from build123d import *

# Parameters (mm, degrees)
F0_R     = 16
F1_DEPTH = 16
F1_TAPER = 1
F2_R     = 16
F3_DEPTH = 16
F4_R     = 2.5
F5_DEPTH = 5
F7_R     = 4.75
F8_DEPTH = 1.5


with BuildPart() as f1:
    # F0 (on Top) → F1 (new body)
    with BuildSketch(Plane.XY):
        Circle(F0_R)
    extrude(amount=F1_DEPTH, taper=F1_TAPER)

    # F2 (on Front) → F3 (cut, symmetric)
    with BuildSketch(Plane.XZ):
        with Locations((0, 20)):
            Circle(F2_R)
    extrude(amount=F3_DEPTH, both=True, mode=Mode.SUBTRACT)

    # F4 (on face) → F5 (cut)
    with BuildSketch(Plane(origin=(0, 0, 0), x_dir=(1, 0, 0), z_dir=(0, 0, -1))):
        Circle(F4_R)
    extrude(amount=-F5_DEPTH, mode=Mode.SUBTRACT)

    # F7 (on offset) → F8 (cut)
    with BuildSketch(Plane.XY.offset(5)):
        Circle(F7_R)
    extrude(amount=-F8_DEPTH, mode=Mode.SUBTRACT)


solid = f1.part
Work out the finished part from the listing and answer in its coordinate system (mm). A direction names the side the tool comes from. Give positions to 0.01 mm unless a question says otherwise; leave off trailing zeros. Order: outer loops, then holes, each group sorted by start corner. A loop starts at its lowest first (then second) coordinate and runs counter-clockwise, first axis right, second up. Notation, with made-up numbers: (60.25, 29) -> (77.25, 29) arc R16 cw to (77.25, 48) -> close; hole circle Ø4 at (-16.75, -1). An arc over 180 degrees is marked (long way). One line per item, written item: value.
Item 1: Flat-ended cylindrical pins translate along their axes: P1, Ø8, axis at x = 11.5, z = 2.5, coming from the -Y side; P2, Ø12, axis at x = 4, y = -7.5, coming from the +Z side; P3, Ø6, axis at x = 8, y = -8, coming from the +Z side. Find the tip coordinate at first contact, or state that the pin passes through.
Answer sheet:
P1: y = -14.09
P2: z = 7.51
P3: z = 8.38
Item 2: A tool of negligible diameter and unlimited length cuts with its end or side. For faces 1 (the flat face through (2, -2, 3.5)), 2 (the cylindrical face through (-4.9, -0.22, 4.77)), from which of +Z, -Z, +X, -X, +Y, -Y can it reach the whole face along a straight path? Write none if from no direction.
Answer sheet:
face 1: +Z
face 2: +Z, +Y, -Y
Item 3: Determine the mould class of faces 3 (the flat face through (0, -3, 0)), 4 (the conical face through (-11.71, 10.74, 6.33)), 5 (the cylindrical face through (-0.54, 2.44, 1.73)) for opening direction X: released by +X, released by -X, zero draft, split by the parting line, or undercut.
Answer sheet:
face 3: zero draft
face 4: split by the parting line
face 5: undercut
Item 4: Find section A-A, the plane z = 11.5. Give the vertices of the cut face in (x, y).
Answer sheet:
outline: (-13.56, -8.12) -> (-13.56, 8.12) arc R15.8 ccw to start; (13.56, -8.12) arc R15.8 ccw to (13.56, 8.12) -> close
Item 5: Straight lines are drawn through the part: probe 1 along Y at (x, z) = (0, 3.8); probe 2 along X at (y, z) = (3, 11.5); probe 3 along Y at (x, z) = (0, 1.5). For each, find the intervals that lie inside material, in ascending order.
Answer sheet:
probe 1: -15.93 to -4.75, 4.75 to 15.93
probe 2: -15.51 to -13.56, 13.56 to 15.51
probe 3: -15.97 to -2.5, 2.5 to 15.97
Item 6: Find section B-B, the plane z = 5.25. Give the vertices of the cut face in (x, y).
Answer sheet:
outline: (-6.2, -14.65) -> (-6.2, 14.65) arc R15.91 ccw to start; (6.2, -14.65) arc R15.91 ccw to (6.2, 14.65) -> close
